Geometry: final body of the model. Coordinates: model frame, mm. A direction names the side the tool comes from. Round coordinates to 2 decimals unless told otherwise and drop trailing zeros. Loops run counter-clockwise (first coordinate to the right, second up) from the corner with the lowest first, then second, coordinate; pieces in that order, holes last. Notation, with made-up numbers: M -26.5,-13.5 L 30.5,-13.5 A5 ccw 30.5,-9.5 Z; hole C 81,-39 d10. An arc over 180 degrees is marked long. Answer as a JSON object with one key per item and string values.
from build123d import *

# Parameters (mm, degrees)
CROQUIS1_W                         = 60
CROQUIS1_H                         = 70
BRIDA_BASE1_DEPTH                  = 1.5
BRIDA_DE_ARISTA1_STRIP_W           = 7.4732
BRIDA_DE_ARISTA1_STRIP_H           = 1.5
BRIDA_DE_ARISTA1_STRIP_CUT_DEPTH   = 70
BRIDA_DE_ARISTA1_STRIP_2_W         = 7.4732
BRIDA_DE_ARISTA1_STRIP_2_H         = 1.5
BRIDA_DE_ARISTA1_STRIP_CUT_2_DEPTH = 70
BRIDA_DE_ARISTA1_DEPTH             = 70
BRIDA_DE_ARISTA1_BEND_DEPTH        = 70
ROMPER_START                       = 36.062445841
ROMPER_ESQUINA1_OUTLINE_W          = 64
ROMPER_ESQUINA1_OUTLINE_H          = 51.062445841
ROMPER_ESQUINA1_DEPTH              = 3.535533905
ROMPER_START_2                     = -13.435028843
ROMPER_ESQUINA1_2_OUTLINE_W        = 64
ROMPER_ESQUINA1_2_OUTLINE_H        = 3.937554159
ROMPER_ESQUINA1_2_DEPTH            = 7.071067812
CROQUIS13_R                        = 2.5
CORTAR_EXTRUIR1_DEPTH              = 73.567210226


# Read off the part's stored shape, not the designer's step: Romper esquina1
# Sheet-metal steps are written as plain solids
with BuildPart() as part:
    # Croquis1 → Brida base1 (new body)
    with BuildSketch(Plane.XY):
        Rectangle(CROQUIS1_W, CROQUIS1_H)
    extrude(amount=-BRIDA_BASE1_DEPTH)

    # Brida de arista1 strip (across the edge) → Brida de arista1 strip cut (cut)
    with BuildSketch(Plane(origin=(30, -35, 0), x_dir=(-1, 0, 0), z_dir=(0, 1, 0))):
        with Locations((-1.5, -0.75)):
            Rectangle(BRIDA_DE_ARISTA1_STRIP_W, BRIDA_DE_ARISTA1_STRIP_H)
    extrude(amount=BRIDA_DE_ARISTA1_STRIP_CUT_DEPTH, mode=Mode.SUBTRACT)

    # Brida de arista1 strip 2 (across the edge) → Brida de arista1 strip cut 2 (cut)
    with BuildSketch(Plane(origin=(-30, 35, 0), x_dir=(1, 0, 0), z_dir=(0, -1, 0))):
        with Locations((-1.5, -0.75)):
            Rectangle(BRIDA_DE_ARISTA1_STRIP_2_W, BRIDA_DE_ARISTA1_STRIP_2_H)
    extrude(amount=BRIDA_DE_ARISTA1_STRIP_CUT_2_DEPTH, mode=Mode.SUBTRACT)

    # Brida de arista1 section (across the edge) → Brida de arista1 (add)
    with BuildSketch(Plane(origin=(30, -35, 0), x_dir=(-1, 0, 0), z_dir=(0, 1, 0))):
        with BuildLine():
            Line((0, 0.7366), (0, 21))
            Line((0, 21), (1.5, 21))
            Line((1.5, 21), (1.5, 0.7366))
            ThreePointArc((1.5, 0.7366), (1.715745145, 0.215745145), (2.2366, 0))
            Line((2.2366, 0), (2.2366, -1.5))
            ThreePointArc((2.2366, -1.5), (0.655084973, -0.844915027), (0, 0.7366))
        make_face()
    extrude(amount=BRIDA_DE_ARISTA1_DEPTH)

    # Brida de arista1 section 2 (across the edge) → Brida de arista1 bend (add)
    with BuildSketch(Plane(origin=(-30, 35, 0), x_dir=(1, 0, 0), z_dir=(0, -1, 0))):
        with BuildLine():
            Line((0, 0.7366), (0, 21))
            Line((0, 21), (1.5, 21))
            Line((1.5, 21), (1.5, 0.7366))
            ThreePointArc((1.5, 0.7366), (1.715745145, 0.215745145), (2.2366, 0))
            Line((2.2366, 0), (2.2366, -1.5))
            ThreePointArc((2.2366, -1.5), (0.655084973, -0.844915027), (0, 0.7366))
        make_face()
    extrude(amount=BRIDA_DE_ARISTA1_BEND_DEPTH)

    # Romper esquina1 outline → Romper esquina1 (cut)
    with BuildSketch(Plane(origin=(0, 0, 0), x_dir=(1, 0, 0), z_dir=(0, 0.707106781186548, 0.707106781186547)).offset(ROMPER_START)):
        with Locations((0, -10.53122292)):
            Rectangle(ROMPER_ESQUINA1_OUTLINE_W, ROMPER_ESQUINA1_OUTLINE_H)
    extrude(amount=ROMPER_ESQUINA1_DEPTH, mode=Mode.SUBTRACT)

    # Romper esquina1 2 outline → Romper esquina1 2 (cut)
    with BuildSketch(Plane(origin=(0, 0, 0), x_dir=(1, 0, 0), z_dir=(0, 0.707106781186548, 0.707106781186547)).offset(ROMPER_START_2)):
        with Locations((0, -38.03122292)):
            Rectangle(ROMPER_ESQUINA1_2_OUTLINE_W, ROMPER_ESQUINA1_2_OUTLINE_H)
    extrude(amount=ROMPER_ESQUINA1_2_DEPTH, mode=Mode.SUBTRACT)

    # Croquis13 → Cortar-Extruir1 (cut, through all)
    with BuildSketch(Plane(origin=(30, 0, 0), x_dir=(0, 0, -1), z_dir=(1, 0, 0))):
        with Locations((-12.5, 20)):
            Circle(CROQUIS13_R)
        with Locations((-12.5, -20)):
            Circle(CROQUIS13_R)
    extrude(amount=-CORTAR_EXTRUIR1_DEPTH, mode=Mode.SUBTRACT)


solid = part.part
1) Ray query, line 1 (Y direction, x = -29.5, z = 12.5); line 2 (X direction, y = 17, z = 1.5); line 3 (Z direction, x = 0, y = -29). Return the intervals inside material, ascending.
Results:
{"line 1": "-35 to -22.5, -17.5 to 17.5, 22.5 to 35", "line 2": "-30 to -28.5, 28.5 to 30", "line 3": "-1.5 to 0"}
2) Reachability of faces 4 (the flat face through (0, 0, 0)), 5 (the cylindrical face through (-29, -18, 14)) from +Z, -Z, +X, -X, +Y, -Y: full face, straight path, thin tool, end or side. Return the list, or none.
Results:
{"face 4": "+Z, +Y, -Y", "face 5": "+X, -X"}
3) Pin query (flat end, axial travel): P1, Ø4, axis at y = 20, z = 12.5, coming from the -X side. Return the tip coordinate at first contact, or that it passes through.
Results:
{"P1": "through"}
4) Section query A-A (z = 12.5). Return the cut outline in (x, y).
Results:
{"outline": "M -30,-35 L -28.5,-35 L -28.5,-22.5 L -30,-22.5 Z; M -30,-17.5 L -28.5,-17.5 L -28.5,17.5 L -30,17.5 Z; M -30,22.5 L -28.5,22.5 L -28.5,35 L -30,35 Z; M 28.5,-35 L 30,-35 L 30,-22.5 L 28.5,-22.5 Z; M 28.5,-17.5 L 30,-17.5 L 30,17.5 L 28.5,17.5 Z; M 28.5,22.5 L 30,22.5 L 30,35 L 28.5,35 Z"}
5) Section query B-B (y = -20). Return the cut outline in (x, z).
Results:
{"outline": "M -30,0.74 A2.24 ccw -27.76,-1.5 L 27.76,-1.5 A2.24 ccw 30,0.74 L 30,10 L 28.5,10 L 28.5,0.74 A0.74 cw 27.76,0 L -27.76,0 A0.74 cw -28.5,0.74 L -28.5,10 L -30,10 Z; M -30,15 L -28.5,15 L -28.5,21 L -30,21 Z; M 28.5,15 L 30,15 L 30,21 L 28.5,21 Z"}
6) Pull-direction query (Z, two-part tool) for faces 1 (the cylindrical face through (29.33, -0.49, -0.86)), 2 (the flat face through (29, 33, 18)), 3 (the cylindrical face through (-29.24, 22.48, 12.83)); classes: +Z half, -Z half, draft (parallel to the pull), parting line (faces both ways), or undercut.
Results:
{"face 1": "-Z half", "face 2": "+Z half", "face 3": "undercut"}
7) Section query C-C (z = 17.5). Return the cut outline in (x, y), and give its area (3 significant figures).
Results:
{"outline": "M -30,-33.5 L -28.5,-33.5 L -28.5,33.5 L -30,33.5 Z; M 28.5,-33.5 L 30,-33.5 L 30,33.5 L 28.5,33.5 Z", "area": "201 mm2"}
8) Section query D-D (z = 4.5). Return the cut outline in (x, y), and give its area (3 significant figures).
Results:
{"outline": "M -30,-35 L -28.5,-35 L -28.5,35 L -30,35 Z; M 28.5,-35 L 30,-35 L 30,35 L 28.5,35 Z", "area": "210 mm2"}
